Check sheet for the drawn part. Datum: minimum x, y, z corner. Units: mm. A direction names the side the tool comes from. Round coordinates to 2 decimals unless told otherwise and drop trailing zeros. Order: outer loops, then holes, each group sorted by start corner. A loop starts at its lowest first (then second) coordinate and runs counter-clockwise, first axis right, second up. Notation, with made-up numbers: (72, -16.5) -> (76, -16.5) arc R30 ccw to (76, 16.5) -> close; hole circle Ø2 at (-34, 19). An arc over 180 degrees is marked (long way). Write item = value, one per line. Start each with the question number.
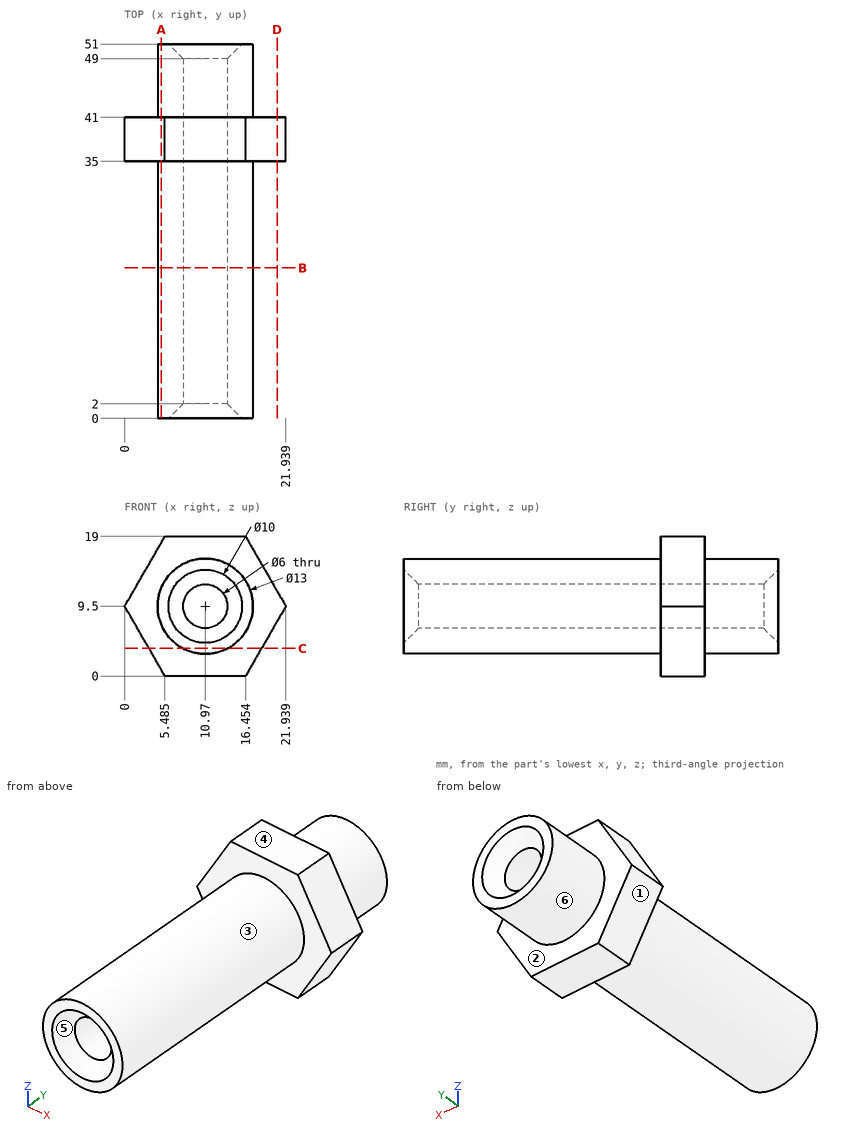
(1) Scan lines: line 1 along X through (y, z) = (39, 9.5); line 2 along X through (y, z) = (16, 9.5); line 3 along Y through (x, z) = (2.75, 12.25). Record each from-to range of solid material in increasing order. Write a range as from..to.
(2) Cross-section at A-A (x = 5). Enter the section's corners in (y, z).
(3) Cross-section at B-B (y = 20.5). Enter the section's corners in (x, z).
(4) Depth check by flat-ended pin: pin 1 (5 mm diameter, centred on y = 22, z = 4.5, fed in from +X); pin 2 (4 mm diameter, centred on x = 4, z = 2.5, fed in from -Y); pin 3 (2 mm diameter, centred on x = 16.5, z = 10.5, fed in from -Y); pin 4 (7 mm diameter, centred on x = 10.97, z = 9.5, fed in from +Y). Enter the tip coordinate at first touch or a pass-through.
(5) Cross-section at C-C (z = 3.75). Enter the section's corners in (x, y).
(6) Set-up check for the marked faces 1, 2 and 3: record each of +Z, -Z, +X, -X, +Y, -Y from which the full face is reachable in a straight line by a thin tool's end or side.
(7) Draft check along Z on the marked faces 4, 5 and 6. Enter one of: +Z half, -Z half, draft (parallel to the pull), parting line (faces both ways), or undercut.
(8) Cross-section at D-D (x = 20.75). Enter the section's corners in (y, z), and give its area (3 significant figures).
Outcome:
q1.line_1 = 0..7.97, 13.97..21.94
q1.line_2 = 4.47..7.97, 13.97..17.47
q1.line_3 = 35..41
q2.outline = (0, 6.93) -> (35, 6.93) -> (35, 0.84) -> (41, 0.84) -> (41, 6.93) -> (51, 6.93) -> (51, 12.07) -> (41, 12.07) -> (41, 18.16) -> (35, 18.16) -> (35, 12.07) -> (0, 12.07) -> close
q3.outline = circle Ø13 at (10.97, 9.5); hole circle Ø6 at (10.97, 9.5)
q4.pin_1 = 16.97
q4.pin_2 = 35
q4.pin_3 = 0
q4.pin_4 = 49.5
q5.outline = (3.32, 35) -> (7.94, 35) -> (7.94, 0) -> (14, 0) -> (14, 35) -> (18.62, 35) -> (18.62, 41) -> (14, 41) -> (14, 51) -> (7.94, 51) -> (7.94, 41) -> (3.32, 41) -> close
q6.face_1 = -Z, -X, +Y, -Y
q6.face_2 = +Y
q6.face_3 = -Y
q7.face_4 = +Z half
q7.face_5 = undercut
q7.face_6 = parting line
q8.outline = (35, 7.44) -> (41, 7.44) -> (41, 11.56) -> (35, 11.56) -> close
q8.area = 24.7 mm^2
